Can you work these out from the model? Positions are in its coordinate system, mm. Face numbers are marked on the shaded views. A direction names the side the tool comes from. Give positions to 0.01 mm unless a question says otherwise; leave off trailing zeros. Loops run counter-clockwise (first coordinate to the right, second up) from the corner with the lowest first, then second, coordinate; pieces in that order, holes last. Notation, with made-up numbers: (57, -13.75) -> (65, -13.75) arc R32 ccw to (65, 18.25) -> close; hole circle Ø6 at (36.5, 55). An arc over 180 degrees is marked (long way). Use CSV: the item, a comma, the result in double quotes.
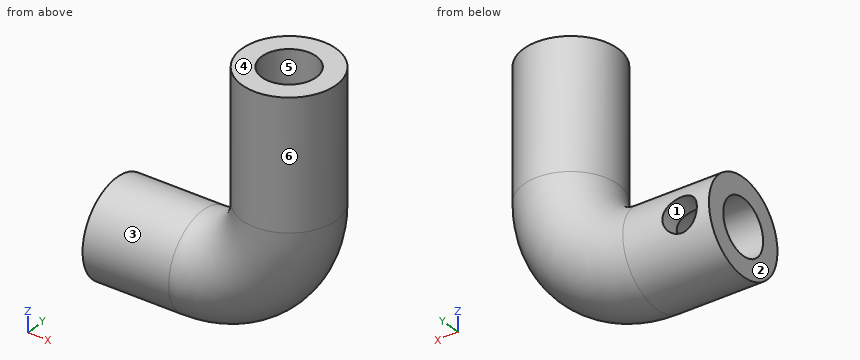
from build123d import *

# Parameters (mm, degrees)
SKETCH4_R           = 5.5
SKETCH6_R           = 3.175
HOLE_SHAFT_DEPTH    = 10
SKETCH7_R           = 3.2
HOLE_POT_DEPTH      = 10
SKETCH8_R           = 2
CUT_EXTRUDE3_DEPTH  = 6.5000001
SKETCH11_W          = 6.737911532
SKETCH11_H          = 1
BOSS_EXTRUDE2_DEPTH = 1


with BuildPart() as part:
    # Sweep2: sweep along a path in PROFILE
    with BuildLine(Plane(origin=(0, 0, 0), x_dir=(1, 0, 0), z_dir=(0, 1, 0))) as sweep2_path:
        Line((2.5, -25), (2.5, -10))
        ThreePointArc((2.5, -10), (-0.428932188, -2.928932188), (-7.5, 0))
        Line((-7.5, 0), (-17.5, 0))
    # Sketch4 → Sweep2 (sweep)
    with BuildSketch(Plane.XY.offset(25)):
        with Locations((2.5, 0)):
            Circle(SKETCH4_R)
    sweep(path=sweep2_path.line)

    # Sketch6 → HOLE_SHAFT (cut)
    with BuildSketch(Plane.XY.offset(25)):
        with Locations((2.5, 0)):
            Circle(SKETCH6_R)
    extrude(amount=-HOLE_SHAFT_DEPTH, mode=Mode.SUBTRACT)

    # Sketch7 → HOLE_POT (cut)
    with BuildSketch(Plane.ZY.offset(17.5)):
        Circle(SKETCH7_R)
    extrude(amount=-HOLE_POT_DEPTH, mode=Mode.SUBTRACT)

    # Sketch8 → Cut-Extrude3 (cut, through all)
    with BuildSketch(Plane(origin=(0, 0, 0), x_dir=(1, 0, 0), z_dir=(0, 1, 0))):
        with Locations((-14.096251262, 0)):
            Circle(SKETCH8_R)
    extrude(amount=CUT_EXTRUDE3_DEPTH, mode=Mode.SUBTRACT)

    # Sketch11 → Boss-Extrude2 (add)
    with BuildSketch(Plane.ZY.offset(7.5)):
        Rectangle(SKETCH11_W, SKETCH11_H)
    extrude(amount=BOSS_EXTRUDE2_DEPTH)


solid = part.part
(1) If we section it at D-D, the plane z = 14.5: Write out the boundary of the cut face in (x, y).
Answer sheet:
outline,"circle Ø11 at (2.5, 0)"
(2) If we section it at B-B, the plane y = 0: Write out the boundary of the cut face in (x, z) (3 decimals).
Answer sheet:
outline,"(-17.5, -5.5) -> (-7.5, -5.5) arc R15.5 ccw to (8, 10) -> (8, 25) -> (5.675, 25) -> (5.675, 15) -> (-0.675, 15) -> (-0.675, 25) -> (-3, 25) -> (-3, 10) arc R4.5 cw to (-7.5, 5.5) -> (-17.5, 5.5) -> (-17.5, 3.2) -> (-8.5, 3.2) -> (-8.5, -3.2) -> (-17.5, -3.2) -> close"
(3) We'd pull the mould along Y, two halves only. Please class the marked faces 4, 5 and 6: released by +Y, released by -Y, zero draft, split by the parting line, or undercut.
Answer sheet:
face 4,"zero draft"
face 5,"undercut"
face 6,"split by the parting line"
(4) If we section it at C-C, the plane x = -9.25: Write out the boundary of the cut face in (y, z), then the cut area to 3 significant figures.
Answer sheet:
outline,"circle Ø11 at (0, 0); hole circle Ø6.4 at (0, 0)"
area,"62.9 mm2"
(5) If we section it at A-A, the plane z = 21.5: Write out the boundary of the cut face in (x, y) (3 decimals).
Answer sheet:
outline,"circle Ø11 at (2.5, 0); hole circle Ø6.35 at (2.5, 0)"
(6) If I drill on L1, parallel to Y at x = 2.5, z = 19.75 (3 decimals); L2, parallel to Y at x = -9.25, z = 4.5; L3, parallel to X at y = 3.9, z = 0, over which ranges is the centre line in solid material (lowest first)? Write a range as from..to.
Answer sheet:
L1,"y = -5.5..-3.175, 3.175..5.5"
L2,"y = -3.16..3.16"
L3,"x = -17.5..-16.1, -12.1..2.12"
(7) Will these pins go through, and if not, where does the flat tip stop? pin 1 Ø5 at (x, y) = (4, 2.5) entering from +Z; pin 2 Ø3 at (x, z) = (5.5, 18.5) entering from -Y; pin 3 Ø4 at (x, y) = (2.5, 0) entering from -Z; pin 4 Ø1 at (x, y) = (-13, 3) entering from -Z.
Answer sheet:
pin 1,"stops at z = 25"
pin 2,"stops at y = -5.29"
pin 3,"stops at z = -3.28"
pin 4,"stops at z = -4.9"
(8) Which directions (+Z, -Z, +X, -X, +Y, -Y) give clear straight access to the entire face, cutting with the end or side of a thin tool? Please do the marked faces 1, 2 and 3.
Answer sheet:
face 1,"+Y"
face 2,"+Z, -Z, -X, +Y, -Y"
face 3,"-X"
